Can you work these out from the model? Positions are in its coordinate system, mm. A direction names the side the tool comes from. Coordinates: 2 decimals unless noted, no trailing zeros. Write each loop counter-clockwise with the first axis right and the second up, starting at its lowest first coordinate (ties: lowest second). Pieces come first, ordered by that corner, then holes. Notation, with made-up numbers: (-38, 65.5) - (9, 65.5) arc R10 cw to (9, 73.5) - close; hole circle Ø5 at (46, 45.25). An arc over 180 degrees is marked (long way). Write each question's results on one line, items separated by ' | '. Start each with the question number.
```python
from build123d import *

# Parameters (mm, degrees)
BOSS_EXTRUDE1_DEPTH = 66
SKETCH4_R           = 15
BOSS_EXTRUDE2_DEPTH = 10
CUT_EXTRUDE2_DEPTH  = 108.615054709
SKETCH5_W           = 16
SKETCH5_H           = 23
CUT_EXTRUDE3_DEPTH  = 128.988280714
SKETCH6_W           = 10
SKETCH6_H           = 10
BOSS_EXTRUDE3_DEPTH = 5
SKETCH7_W           = 12
SKETCH7_H           = 12
BOSS_EXTRUDE4_DEPTH = 5
CUT_EXTRUDE4_DEPTH  = 3


with BuildPart() as part:
    # Sketch2 → Boss-Extrude1 (new body)
    with BuildSketch(Plane.XY):
        with BuildLine():
            ThreePointArc((65, 0), (38.160843726, 29.198871234), (-1.89e-07, 40))
            ThreePointArc((-1.89e-07, 40), (-38.160843886, 29.198871136), (-65, 0))
            Line((-65, 0), (-65, -40))
            Line((-65, -40), (65, -40))
            Line((65, -40), (65, 0))
        make_face()
    extrude(amount=BOSS_EXTRUDE1_DEPTH)

    # Sketch4 → Boss-Extrude2 (add)
    with BuildSketch(Plane(origin=(65, 0, 0), x_dir=(0, 0, -1), z_dir=(1, 0, 0))):
        with Locations(Location((-33, -20, 0), (0, 0, 90))):
            Circle(SKETCH4_R)
    extrude(amount=BOSS_EXTRUDE2_DEPTH)

    # Sketch3 → Cut-Extrude2 (cut, through all)
    with BuildSketch(Plane.XY.offset(66)):
        with BuildLine():
            Line((-25, 5), (23, 5))
            ThreePointArc((23, 5), (30.071067812, 2.071067812), (33, -5))
            Line((33, -5), (33, -40))
            Line((33, -40), (-35, -40))
            Line((-35, -40), (-35, -5))
            ThreePointArc((-35, -5), (-32.071067812, 2.071067812), (-25, 5))
        make_face()
    extrude(amount=-CUT_EXTRUDE2_DEPTH, mode=Mode.SUBTRACT)

    # Sketch5 → Cut-Extrude3 (cut, through all)
    with BuildSketch(Plane.XZ.offset(40)):
        with Locations((-57, 54.5)):
            Rectangle(SKETCH5_W, SKETCH5_H)
        with Locations((-57, 11.5)):
            Rectangle(SKETCH5_W, SKETCH5_H)
    extrude(amount=-CUT_EXTRUDE3_DEPTH, mode=Mode.SUBTRACT)

    # Sketch6 → Boss-Extrude3 (add)
    with BuildSketch(Plane.XZ.offset(40)):
        with Locations((-48.5, 33)):
            Rectangle(SKETCH6_W, SKETCH6_H)
    extrude(amount=BOSS_EXTRUDE3_DEPTH)

    # Sketch7 → Boss-Extrude4 (add)
    with BuildSketch(Plane.XZ.offset(40)):
        with Locations((41.5, 13.9)):
            Rectangle(SKETCH7_W, SKETCH7_H)
        with Locations((41.5, 52.1)):
            Rectangle(SKETCH7_W, SKETCH7_H)
    extrude(amount=BOSS_EXTRUDE4_DEPTH)

    # Sketch8 → Cut-Extrude4 (cut)
    with BuildSketch(Plane(origin=(75, 0, 0), x_dir=(0, 0, -1), z_dir=(1, 0, 0))):
        with BuildLine():
            Line((-40.689709202, -10.145134583), (-35, -20))
            Line((-35, -20), (-40.689709202, -29.854865417))
            ThreePointArc((-40.689709202, -29.854865417), (-33, -32.5), (-25.310290798, -29.854865417))
            Line((-25.310290798, -29.854865417), (-31, -20))
            Line((-31, -20), (-25.310290798, -10.145134583))
            ThreePointArc((-25.310290798, -10.145134583), (-33, -7.5), (-40.689709202, -10.145134583))
        make_face()
        with BuildLine():
            Line((-36.154700538, -20), (-41.464916663, -10.802435872))
            ThreePointArc((-41.464916663, -10.802435872), (-45.5, -20), (-41.464916663, -29.197564128))
            Line((-41.464916663, -29.197564128), (-36.154700538, -20))
        make_face()
        with BuildLine():
            ThreePointArc((-24.535083337, -29.197564128), (-20.5, -20), (-24.535083337, -10.802435872))
            Line((-24.535083337, -10.802435872), (-29.845299462, -20))
            Line((-29.845299462, -20), (-24.535083337, -29.197564128))
        make_face()
    extrude(amount=-CUT_EXTRUDE4_DEPTH, mode=Mode.SUBTRACT)


solid = part.part
```
Q1. Thinking about a two-plate mould opening in Y: for faces 1 (the face through (73.521, -15.337, 27.153)), 2 (the face through (41, -42, 58.1)), which applies, pulls with the +Y half, pulls with the -Y half, needs draft (parallel to the pull), parting line crosses it, or undercut?
Q2. If we section it at B-B (y = -2): Please give me the cut outline in (x, z).
Q3. For faces 3 (the face through (-57, -17, 43)), 4 (the face through (33, -22, 33)), 5 (the face through (72, -20, 24)), 6 (the face through (47.5, -42, 52)), 7 (the face through (35.5, -42, 14)), which set-ups out of +Z, -Z, +X, -X, +Y, -Y let a thin tool reach every point of the face, with its end or its side?
Q4. If we section it at D-D (y = 11): Please give me the cut outline in (x, z).
Q5. If we section it at C-C (x = 37.5): Please give me the cut outline in (y, z).
Q6. I need wall thicknesses on line 1 along X through (y, z) = (-16.5, 45.5); line 2 along X through (y, z) = (-30, 37.5); line 3 along Z through (x, y) = (-55.5, -9.5). Which ranges of each line are inside material? Lowest first, please. Write a range as from..to.
Q7. I'm going to push flat-ended pins straight in: pin 1 Ø5.5 at (x, y) = (41, -43.5) entering from -Z; pin 2 Ø5.5 at (y, z) = (-42, 32.5) entering from +X; pin 3 Ø3 at (x, z) = (22, 30.5) entering from +Y. Where does each tip first touch, or does it pass through?
Q8. If we section it at A-A (z = 33): Please give me the cut outline in (x, y) (1 decimal), then the cut area to 3 significant figures.
Answer list:
1) face 1: undercut | face 2: needs draft
2) outline: (-65, 23) - (-49, 23) - (-49, 0) - (-34.54, 0) - (-34.54, 66) - (-49, 66) - (-49, 43) - (-65, 43) - close; (32.54, 0) - (65, 0) - (65, 66) - (32.54, 66) - close
3) face 3: +Z, -X, +Y, -Y | face 4: +Z, -Z, -Y | face 5: +X | face 6: +Z, -Z, +X, -Y | face 7: +Z, -Z, -X, -Y
4) outline: (-58.16, 23) - (-49, 23) - (-49, 0) - (58.16, 0) - (58.16, 66) - (-49, 66) - (-49, 43) - (-58.16, 43) - close
5) outline: (-45, 7.9) - (-40, 7.9) - (-40, 0) - (29.6, 0) - (29.6, 66) - (-40, 66) - (-40, 58.1) - (-45, 58.1) - (-45, 46.1) - (-40, 46.1) - (-40, 19.9) - (-45, 19.9) - close
6) line 1: x = -49..-35, 33..75 | line 2: x = -65..-35, 33..72 | line 3: z = 23..43
7) pin 1: stops at z = 7.9 | pin 2: stops at x = 65 | pin 3: stops at y = 37.05
8) outline: (-65, -40) - (-53.5, -40) - (-53.5, -45) - (-43.5, -45) - (-43.5, -40) - (-35, -40) - (-35, -5) arc R10 cw to (-25, 5) - (23, 5) arc R10 cw to (33, -5) - (33, -40) - (65, -40) - (65, -35) - (75, -35) - (75, -32.5) - (72, -32.5) - (72, -7.5) - (75, -7.5) - (75, -5) - (65, -5) - (65, 0) arc R72.8 ccw to (-65, 0) - close | area: 6,170 mm2
